from build123d import *
from build123d.topology import SkipClean

# Parameters (mm, degrees)
EXTRUDE_1_DEPTH          = 20
EXTRUDE_2_DEPTH          = 8
EXTRUDE_3_DEPTH          = 11
CUT_EXTRUDE_7_DEPTH      = 35.292856399
CUT_EXTRUDE_7_DEPTH_BACK = 35.292856399


with BuildPart() as part:
    # 草图2 → 凸台-拉伸1 (new body)
    with BuildSketch(Plane(origin=(0, 0, 0), x_dir=(1, 0, 0), z_dir=(0, 1, 0))):
        with BuildLine():
            ThreePointArc((26, 0), (23.071067812, 7.071067812), (16, 10))
            ThreePointArc((16, 10), (6, 0), (16, -10))
            ThreePointArc((16, -10), (23.071067812, -7.071067812), (26, 0))
        make_face()
    extrude(amount=EXTRUDE_1_DEPTH)

    # 草图2<3> → 凸台-拉伸2 (add)
    with BuildSketch(Plane(origin=(0, 0, 0), x_dir=(1, 0, 0), z_dir=(0, 1, 0))):
        with BuildLine():
            Line((16, 10), (-16, 10))
            ThreePointArc((-16, 10), (-26, 0), (-16, -10))
            Line((-16, -10), (16, -10))
            ThreePointArc((16, -10), (6, 0), (16, 10))
        make_face()
    extrude(amount=EXTRUDE_2_DEPTH)

    # 草图7 → 凸台-拉伸3 (add)
    with BuildSketch(Plane(origin=(0, 0, 0), x_dir=(1, 0, 0), z_dir=(0, 1, 0))):
        with BuildLine():
            Line((-16, 5), (-2, 5))
            ThreePointArc((-2, 5), (3, 0), (-2, -5))
            Line((-2, -5), (-16, -5))
            ThreePointArc((-16, -5), (-21, 0), (-16, 5))
        make_face()
        with BuildLine():
            Line((-16, 3), (-2, 3))
            ThreePointArc((-2, 3), (1, 0), (-2, -3))
            Line((-2, -3), (-16, -3))
            ThreePointArc((-16, -3), (-19, 0), (-16, 3))
        make_face(mode=Mode.SUBTRACT)
    extrude(amount=EXTRUDE_3_DEPTH)

    # 草图7<6> → 切除-拉伸7 (cut, two sides: drawn at the far end of the back side and taken through both)
    with SkipClean():  # the faces are left unmerged after this step: merging them gives an invalid solid
        with BuildSketch(Plane(origin=(0, 0, 0), x_dir=(1, 0, 0), z_dir=(0, 1, 0)).offset(-CUT_EXTRUDE_7_DEPTH_BACK)):
            with BuildLine():
                Line((-16, -3), (-2, -3))
                ThreePointArc((-2, -3), (1, 0), (-2, 3))
                Line((-2, 3), (-16, 3))
                ThreePointArc((-16, 3), (-19, 0), (-16, -3))
            make_face()
        extrude(amount=CUT_EXTRUDE_7_DEPTH + CUT_EXTRUDE_7_DEPTH_BACK, mode=Mode.SUBTRACT)
    add(part.part.scale(1), mode=Mode.REPLACE)  # the faces are merged on a copy

    # 草图13 → Ø1.0mm 暗销孔1 (revolve, cut)
    with BuildSketch(Plane(origin=(16.218423998, 20, 0), x_dir=(0, 0, 1), z_dir=(1, 0, 0))):
        Polygon((0, 0), (0, 20), (7, 20), (7, 0), (0.525, 0), align=None)
    revolve(axis=Axis((16.218423998, 26.35, 0), (0, -1, 0)), mode=Mode.SUBTRACT)


solid = part.part
The model under review builds one solid part; all positions refer to its coordinate system, in mm. A direction names the side the tool comes from. Round coordinates to 2 decimals unless told otherwise and drop trailing zeros. Write each loop counter-clockwise with the first axis right and the second up, starting at its lowest first coordinate (ties: lowest second). Pieces come first, ordered by that corner, then holes. Notation, with made-up numbers: M 31,68 L 83,68 A5 ccw 83,76 Z; hole C 26.5,79.25 d7. An arc over 180 degrees is marked long. Answer as CSV lines item,"result". Start each with the question number.
Q1. Consider section B-B, the plane x = -8. Give the boundary of the cut face in (y, z).
Q2. Consider section C-C, the plane x = 4. Give the boundary of the cut face in (y, z).
Q3. Consider section D-D, the plane y = 18.75. Give the boundary of the cut face in (x, z), then the cut area to 3 significant figures.
Q4. Consider section A-A, the plane x = 22.5. Give the boundary of the cut face in (y, z), then the cut area to 3 significant figures.
Q5. Wall thickness on line 1 along X through (y, z) = (9.25, 0); line 2 along X through (y, z) = (4.25, 0); line 3 along X through (y, z) = (13.75, 0): over which ranges is each line inside the solid? List them lowest first.
Q6. Clearance check with flat-ended pins moving along their axes: P1, Ø2.5, axis at x = -7.5, y = 10, coming from the -Z side; P2, Ø2.5, axis at x = -9, y = 9.5, coming from the +Z side; P3, Ø11, axis at x = -7, z = 1.5, coming from the +Y side. State where each tip first meets the part, or that it passes through.
Q7. The part is to be moulded in two halves that separate along Z. For faces 4 (the face through (0, 4, 10)), 5 (the face through (1, 5, 0)), 6 (the face through (0.4, 0, 2.1)), say which applies: +Z half, -Z half, draft (parallel to the pull), parting line (faces both ways), or undercut.
Q8. Tool access review of faces 1 (the face through (-10, 8, -7)), 2 (the face through (-9, 9, -5)), 3 (the face through (-9, 5, -3)): name each direction out of +Z, -Z, +X, -X, +Y, -Y from which nothing blocks a thin tool from reaching the whole face with its end or side.
Result set:
1,outline,"M 0,-10 L 8,-10 L 8,-5 L 11,-5 L 11,-3 L 0,-3 Z; M 0,3 L 11,3 L 11,5 L 8,5 L 8,10 L 0,10 Z"
2,outline,"M 0,-10 L 8,-10 L 8,10 L 0,10 Z"
3,outline,"C 16,0 d20; hole C 16.22,0 d14"
3,area,"160 mm²"
4,outline,"M 0,-7.6 L 20,-7.6 L 20,-3.09 L 0,-3.09 Z; M 0,3.09 L 20,3.09 L 20,7.6 L 0,7.6 Z"
4,area,"180 mm²"
5,line 1,"x = -21 to -19, 1 to 3, 6 to 9.22, 23.22 to 26"
5,line 2,"x = -26 to -19, 1 to 9.22, 23.22 to 26"
5,line 3,"x = 6 to 9.22, 23.22 to 26"
6,P1,"stops at z = -5"
6,P2,"stops at z = 5"
6,P3,"stops at y = 11"
7,face 4,"+Z half"
7,face 5,"undercut"
7,face 6,"draft"
8,face 1,"+Y"
8,face 2,"-Z, -X, +Y"
8,face 3,"+Y, -Y"
